from build123d import *

# Parameters (mm, degrees)
F1_DEPTH = 7
F2_W     = 5.193473
F2_H     = 5
F3_DEPTH = 25
F4_R     = 0.75
F5_DEPTH = 25


with BuildPart() as f1:
    # F0 (on Front) → F1 (new body)
    with BuildSketch(Plane.XZ):
        with BuildLine():
            Line((30, 5), (0, 5))
            ThreePointArc((0, 5), (-5, 0), (0, -5))
            Line((0, -5), (30, -5))
            ThreePointArc((30, -5), (35, 0), (30, 5))
        make_face()
    extrude(amount=F1_DEPTH)

    # F2 (on face) → F3 (cut)
    with BuildSketch(Plane.XY.offset(5)):
        with Locations((32.596736, -3.5)):
            Rectangle(F2_W, F2_H)
    extrude(amount=-F3_DEPTH, mode=Mode.SUBTRACT)

    # F4 (on face) → F5 (cut)
    with BuildSketch(Plane.XZ.offset(7)):
        with Locations((32.5, 0)):
            Circle(F4_R)
        with Locations((-2.5, 0)):
            Circle(F4_R)
    extrude(amount=-F5_DEPTH, mode=Mode.SUBTRACT)


solid = f1.part
Design review of the part built by this model. Coordinates are the model's own, in mm. A direction names the side the tool comes from. Give positions to 0.01 mm unless a question says otherwise; leave off trailing zeros. Loops run counter-clockwise (first coordinate to the right, second up) from the corner with the lowest first, then second, coordinate; pieces in that order, holes last. Notation, with made-up numbers: (-32.75, 2) - (5.25, 2) arc R16 cw to (5.25, 32) - close; hole circle Ø7 at (37, 57). An arc over 180 degrees is marked (long way). Write item = value, one per line.
1) Take a section at B-B on x = 32.5. State the section outline as (y, z) points, and give its area (3 significant figures).
Result sheet:
outline = (-7, -4.33) - (-6, -4.33) - (-6, -0.75) - (-7, -0.75) - close; (-7, 0.75) - (-6, 0.75) - (-6, 4.33) - (-7, 4.33) - close; (-1, -4.33) - (0, -4.33) - (0, -0.75) - (-1, -0.75) - close; (-1, 0.75) - (0, 0.75) - (0, 4.33) - (-1, 4.33) - close
area = 14.3 mm2
2) Take a section at A-A on z = 0. State the section outline as (x, y) points.
Result sheet:
outline = (-5, -7) - (-3.25, -7) - (-3.25, 0) - (-5, 0) - close; (-1.75, -7) - (31.75, -7) - (31.75, -6) - (30, -6) - (30, -1) - (31.75, -1) - (31.75, 0) - (-1.75, 0) - close; (33.25, -7) - (35, -7) - (35, -6) - (33.25, -6) - close; (33.25, -1) - (35, -1) - (35, 0) - (33.25, 0) - close
3) To check wall thickness, follow line 1 (X direction, y = -6.5, z = 0.5); line 2 (Z direction, x = -2.5, y = -4); line 3 (Z direction, x = -2, y = -4). State the ranges of each line that lie inside material, in increasing order.
Result sheet:
line_1 = -4.97 to -3.06, -1.94 to 31.94, 33.06 to 34.97
line_2 = -4.33 to -0.75, 0.75 to 4.33
line_3 = -4.58 to -0.56, 0.56 to 4.58
4) Draft analysis for pull direction X (two halves, no side actions). For faces 1 (the face through (33.215, -0.507, 0.225)), 2 (the face through (15, 0, 0)), 3 (the face through (35, -6.5, -0.1)), state which applies: +X half, -X half, draft (parallel to the pull), parting line (faces both ways), or undercut.
Result sheet:
face_1 = undercut
face_2 = draft
face_3 = +X half
5) Clearance check with flat-ended pins moving along their axes: pin 1 Ø1.5 at (y, z) = (-1, -3) entering from -X; pin 2 Ø2.5 at (y, z) = (-4, -1) entering from +X. State where each tip first meets the part, or that it passes through.
Result sheet:
pin_1 = -4.47
pin_2 = 30
6) Take a section at D-D on x = -2.5. State the section outline as (y, z) points, and give its area (3 significant figures).
Result sheet:
outline = (-7, -4.33) - (0, -4.33) - (0, -0.75) - (-7, -0.75) - close; (-7, 0.75) - (0, 0.75) - (0, 4.33) - (-7, 4.33) - close
area = 50.1 mm2
7) Tool access review of faces 4 (the face through (-3.095, -3.549, -0.456)), 5 (the face through (31, -1, 0)): name each direction out of +Z, -Z, +X, -X, +Y, -Y from which nothing blocks a thin tool from reaching the whole face with its end or side.
Result sheet:
face_4 = +Y, -Y
face_5 = +Z, -Z, +X
8) Take a section at C-C on y = -1.75. State the section outline as (x, z) points, and give its area (3 significant figures).
Result sheet:
outline = (0, -5) - (30, -5) - (30, 5) - (0, 5) arc R5 ccw to start; hole circle Ø1.5 at (-2.5, 0)
area = 338 mm2
